Part model, mm, in its own coordinate system. Give positions to 0.01 mm unless a question says otherwise; leave off trailing zeros. Order: outer loops, then holes, each group sorted by start corner. A loop starts at its lowest first (then second) coordinate and runs counter-clockwise, first axis right, second up.
1. Slice it at B-B on z = 0. List the corners of the cut face in (x, y).
2. Slice it at D-D on x = 112.5. List the corners of the cut face in (y, z), and give its area (3 significant figures).
3. Drop flat-ended pins along their axis: pin 1 Ø2 at (x, z) = (64, 16) entering from -Y; pin 2 Ø16.5 at (x, z) = (11.5, 5.5) entering from +Y. Give the stop position or say it passes through.
4. Slice it at A-A on y = -1.1. List the corners of the cut face in (x, z).
5. Probe line 1 (Z direction, x = 76, y = -1.45); line 2 (X direction, y = -3.1, z = -74); line 3 (Y direction, x = 44, z = 74.5). List the from-to ranges inside material, lowest first.
6. Slice it at C-C on x = 0. List the corners of the cut face in (y, z).
from build123d import *

# Parameters (mm, degrees)
F0_W     = 317.5
F0_H     = 215.9
F1_DEPTH = 3.81
F2_R     = 5.08
F3_R     = 5.08
F4_W     = 279.4
F4_H     = 177.8
F5_DEPTH = 25.4
F6_W     = 279.4
F6_H     = 177.8
F7_DEPTH = 0.254
F8_R     = 27.6352
F9_DEPTH = 0.0635


with BuildPart() as f1:
    # F0 (on Front) → F1 (new body)
    with BuildSketch(Plane.XZ):
        Rectangle(F0_W, F0_H)
    extrude(amount=F1_DEPTH)

    # F2
    f2_edges = [f1.edges().sort_by_distance(p)[0] for p in [
        (-158.75, -1.905, -107.95),
    ]]
    fillet(f2_edges, radius=F2_R)

    # F3
    f3_edges = [f1.edges().sort_by_distance(p)[0] for p in [
        (-158.75, -1.905, 107.95),
        (158.75, -1.905, 107.95),
        (158.75, -1.905, -107.95),
    ]]
    fillet(f3_edges, radius=F3_R)

    # F4 (on face) → F5 (cut)
    with BuildSketch(Plane.XZ.offset(3.81)):
        Rectangle(F4_W, F4_H)
    extrude(amount=-F5_DEPTH, mode=Mode.SUBTRACT)

    # F6 (on face) → F7 (join)
    with BuildSketch(Plane.XZ):
        Rectangle(F6_W, F6_H)
    extrude(amount=F7_DEPTH)

    # F8 (on face) → F9 (cut, symmetric)
    with BuildSketch(Plane.XZ):
        Circle(F8_R)
    extrude(amount=F9_DEPTH, both=True, mode=Mode.SUBTRACT)


solid = f1.part
Data:
1. outline: (-158.75, -3.81) - (-139.7, -3.81) - (-139.7, -0.25) - (139.7, -0.25) - (139.7, -3.81) - (158.75, -3.81) - (158.75, 0) - (27.64, 0) - (27.64, -0.06) - (-27.64, -0.06) - (-27.64, 0) - (-158.75, 0) - close
2. outline: (-3.81, -107.95) - (0, -107.95) - (0, 107.95) - (-3.81, 107.95) - (-3.81, 88.9) - (-0.25, 88.9) - (-0.25, -88.9) - (-3.81, -88.9) - close
2. area: 190 mm2
3. pin 1: stops at y = -0.25
3. pin 2: stops at y = -0.06
4. outline: (-158.75, -102.87) arc R5.08 ccw to (-153.67, -107.95) - (153.67, -107.95) arc R5.08 ccw to (158.75, -102.87) - (158.75, 102.87) arc R5.08 ccw to (153.67, 107.95) - (-153.67, 107.95) arc R5.08 ccw to (-158.75, 102.87) - close; hole (-139.7, -88.9) - (139.7, -88.9) - (139.7, 88.9) - (-139.7, 88.9) - close
5. line 1: z = -107.95 to -88.9, 88.9 to 107.95
5. line 2: x = -158.75 to -139.7, 139.7 to 158.75
5. line 3: y = -0.25 to 0
6. outline: (-3.81, -107.95) - (0, -107.95) - (0, -27.64) - (-0.06, -27.64) - (-0.06, 27.64) - (0, 27.64) - (0, 107.95) - (-3.81, 107.95) - (-3.81, 88.9) - (-0.25, 88.9) - (-0.25, -88.9) - (-3.81, -88.9) - close
